Autodesk Inventor part; units mm, degrees
ref_plane "YZ Plane" through (0, 0, 0) normal (1, 0, 0) x (0, 1, 0)
ref_plane "XZ Plane" through (0, 0, 0) normal (0, 1, 0) x (-1, 0, 0)
ref_plane "XY Plane" through (0, 0, 0) normal (0, 0, 1) x (1, 0, 0)
sketch "Sketch1" plane through (0, 0, 0) normal (0, 0, 1) x (1, 0, 0)
  line L0 (0, 0) -> (100, 0)
  line L1 (100, 0) -> (100, 500)
  line L2 (0, 500) -> (0, 0)
  line L3 (0, 500) -> (17.6777, 482.3223)
  line L4 (100, 500) -> (82.3223, 482.3223)
  line L5 (17.6777, 482.3223) -> (82.3223, 482.3223)
  line L6 (50, -100) -> (-150, -100)
revolve "Revolution1" add sketch "Sketch1" angle 360 about axis through (50, -100, 0) along (-1, 0, 0)
sketch "Sketch2" plane through (100, -100, 0) normal (1, 0, 0) x (0, 0, -1)
  circle A0 centre (0, 0) radius 600
  circle A1 centre (0, 350) radius 37.5
  circle A2 centre (0, 0) radius 100
  circle A3 centre (-350, 0) radius 37.5
  circle A4 centre (0, -350) radius 37.5
  circle A5 centre (350, 0) radius 37.5
  point P0 (0, 100)
  dimension "d8" = 360
extrude "Extrusion1" cut sketch "Sketch2" against normal blind 100 contours A1 | A3 | A4 | A5
thicken "Thicken1" operation add thickness 10 both sides no extend neighbours no toward (1, 0, 0) faces at (100, -364.9419, 262.9039)
thicken "Thicken2" operation add thickness 10 both sides no extend neighbours no toward (-1, 0, 0) faces at (0, -364.9419, 262.9039)
sketch "Sketch3" plane through (110, -100, 0) normal (1, 0, 0) x (0, 0, -1)
  line L0 (-25, 125) -> (25, 125)
  line L1 (25, 125) -> (25, 96.8246)
  line L2 (-25, 96.8246) -> (-25, 125)
  line L3 (-25, 125) -> (0, 100) construction
  line L4 (25, 125) -> (0, 100) construction
  arc A0 (25, 96.8246) -> (-25, 96.8246) centre (0, 0) ccw
  point P0 (0, 100)
extrude "Extrusion2" cut sketch "Sketch3" against normal blind 120
properties part number "Polea-1021920"
Geometry: final body of the model. Coordinates: model frame, mm. A direction names the side the tool comes from. Coordinates: 2 decimals unless noted, no trailing zeros. Order: outer loops, then holes, each group sorted by start corner. A loop starts at its lowest first (then second) coordinate and runs counter-clockwise, first axis right, second up.
(1) First-contact query: pin 1 (4 mm diameter, centred on x = 92, z = -461.5, fed in from -Y); pin 2 (10 mm diameter, centred on x = 22.5, z = -226, fed in from -Y); pin 3 (4 mm diameter, centred on x = 21.5, z = 350.5, fed in from -Y); pin 4 (12 mm diameter, centred on y = 357, z = 390.5, fed in from -X). Flat tips, straight axial feed; report the tip coordinate or a pass-through.
(2) Section query B-B (y = -100). Return the cut outline in (x, z).
(3) Material intervals for probe 1 along Y at (x, z) = (42.5, 0); probe 2 along Y at (x, z) = (81.5, 350); probe 3 along Y at (x, z) = (64, 11), sorted ascending.
(4) Section query C-C (x = 61). Return the cut outline in (y, z).
(5) Section query A-A (z = 0). Return the cut outline in (x, y), plus the area to 3 significant figures.
(6) Draft query along Y for faces 1 (the face through (50.84, -74.656, -322.361)), 2 (the face through (-10, -108, 125)), 3 (the face through (50.84, -199.92, 4.04)), 4 (the face through (16.572, -226.476, 569.554)). Return one class per face: pulls with the +Y half, pulls with the -Y half, needs draft (parallel to the pull), parting line crosses it, or undercut.
(7) Access query for faces 5 (the face through (110, -108, 125)), 6 (the face through (50.453, -226.236, -568.475)), 7 (the face through (51, 25, 0)). Directions: +Z, -Z, +X, -X, +Y, -Y. A direction counts if a zero-diameter tool reaches every point of the face in a straight line with its end or side. Return the directions, or none.
Solution:
1. pin 1: stops at y = -474.81
1. pin 2: stops at y = -638.76
1. pin 3: stops at y = -566.53
1. pin 4: stops at x = -10
2. outline: (-10, -600) - (0, -600) - (17.68, -582.32) - (82.32, -582.32) - (100, -600) - (110, -600) - (110, -387.5) - (-10, -387.5) - close; (-10, -312.5) - (110, -312.5) - (110, -100) - (-10, -100) - close; (-10, 100) - (110, 100) - (110, 312.5) - (-10, 312.5) - close; (-10, 387.5) - (110, 387.5) - (110, 600) - (100, 600) - (82.32, 582.32) - (17.68, 582.32) - (0, 600) - (-10, 600) - close
3. probe 1: y = -682.32 to -487.5, -412.5 to -200, 25 to 212.5, 287.5 to 482.32
3. probe 2: y = -565.4 to -137.5, -62.5 to 365.4
3. probe 3: y = -682.22 to -485.85, -414.15 to -199.39, 25 to 214.15, 285.85 to 482.22
4. outline: circle Ø1164.64 at (-100, 0); hole circle Ø75 at (-450, 0); hole circle Ø75 at (-100, -350); hole circle Ø75 at (-100, 350); hole (-3.18, -25) - (25, -25) - (25, 25) - (-3.18, 25) arc R100 ccw (long way) to start; hole circle Ø75 at (250, 0)
5. outline: (-10, -700) - (0, -700) - (17.68, -682.32) - (82.32, -682.32) - (100, -700) - (110, -700) - (110, -487.5) - (-10, -487.5) - close; (-10, -412.5) - (110, -412.5) - (110, -200) - (-10, -200) - close; (-10, 25) - (110, 25) - (110, 212.5) - (-10, 212.5) - close; (-10, 287.5) - (110, 287.5) - (110, 500) - (100, 500) - (82.32, 482.32) - (17.68, 482.32) - (0, 500) - (-10, 500) - close
5. area: 96,100 mm2
6. face 1: undercut
6. face 2: needs draft
6. face 3: undercut
6. face 4: parting line crosses it
7. face 5: +Z, -Z, +X, +Y, -Y
7. face 6: none
7. face 7: +X, -X
